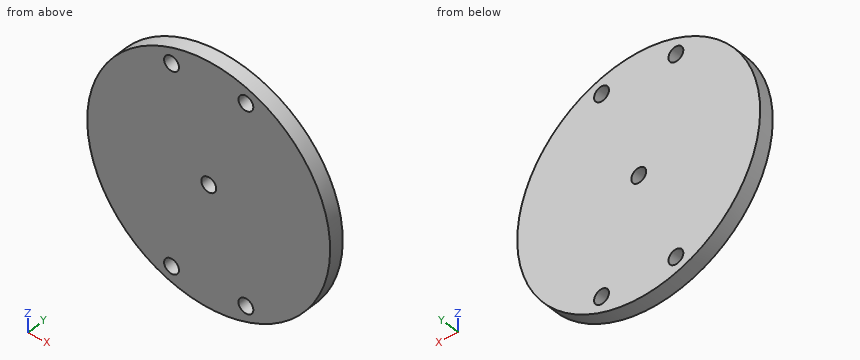
from build123d import *

# Parameters (mm, degrees)
SKETCH1_R           = 49
BOSS_EXTRUDE1_DEPTH = 6
SKETCH2_R           = 3
CUT_EXTRUDE1_DEPTH  = 6


with BuildPart() as part:
    # Sketch1 → Boss-Extrude1 (new body)
    with BuildSketch(Plane(origin=(0, 0, 0), x_dir=(1, 0, 0), z_dir=(0, 1, 0))):
        with Locations(Location((0, 0, 0), (0, 0, 270))):
            Circle(SKETCH1_R)
    extrude(amount=BOSS_EXTRUDE1_DEPTH)

    # Sketch2 → Cut-Extrude1 (cut)
    with BuildSketch(Plane(origin=(0, 6, 0), x_dir=(1, 0, 0), z_dir=(0, 1, 0))):
        with Locations(Location((-15, 40.298883359, 0), (0, 0, 270))):
            Circle(SKETCH2_R)
        with Locations(Location((15, 40.298883359, 0), (0, 0, 270))):
            Circle(SKETCH2_R)
        with Locations(Location((0, 0, 0), (0, 0, 270))):
            Circle(SKETCH2_R)
        with Locations(Location((15, -40.298883359, 0), (0, 0, 270))):
            Circle(SKETCH2_R)
        with Locations(Location((-15, -40.298883359, 0), (0, 0, 270))):
            Circle(SKETCH2_R)
    extrude(amount=-CUT_EXTRUDE1_DEPTH, mode=Mode.SUBTRACT)


solid = part.part
Could you check a few things on this model? Use its own coordinates, in mm. Coordinates: 2 decimals unless noted, no trailing zeros. Order: outer loops, then holes, each group sorted by start corner. A loop starts at its lowest first (then second) coordinate and runs counter-clockwise, first axis right, second up.
Q1. Suppose I cut it at C-C on y = 2.4. Please give me the cut outline in (x, z).
Q2. Will these pins go through, and if not, where does the flat tip stop? pin 1 (2 mm diameter, centred on y = 2, z = 3.5, fed in from +X); pin 2 (5 mm diameter, centred on x = -20, z = 20.5, fed in from -Y); pin 3 (2 mm diameter, centred on x = -13, y = 3.5, fed in from +Z); pin 4 (2 mm diameter, centred on x = -3.5, y = 2, fed in from +Z).
Q3. Suppose I cut it at A-A on x = 0. Please give me the cut outline in (y, z).
Q4. Please list where these lines run through material, in increasing order: L1, parallel to X at y = 2.2, z = -40; L2, parallel to Z at x = -13, y = 5.7; L3, parallel to X at y = 1.15, z = -41.
Q5. Suppose I cut it at D-D on z = 21.5. Please give me the cut outline in (x, y).
Q6. Suppose I cut it at B-B on x = -15. Please give me the cut outline in (y, z), and give its area (3 significant figures).
Answer:
1. outline: circle Ø98 at (0, 0); hole circle Ø6 at (-15, -40.3); hole circle Ø6 at (-15, 40.3); hole circle Ø6 at (0, 0); hole circle Ø6 at (15, -40.3); hole circle Ø6 at (15, 40.3)
2. pin 1: stops at x = 48.94
2. pin 2: stops at y = 0
2. pin 3: stops at z = 47.51
2. pin 4: stops at z = 48.94
3. outline: (0, -49) - (6, -49) - (6, -3) - (0, -3) - close; (0, 3) - (6, 3) - (6, 49) - (0, 49) - close
4. L1: x = -28.3 to -17.99, -12.01 to 12.01, 17.99 to 28.3
4. L2: z = -47.24 to -42.53, -38.06 to 38.06, 42.53 to 47.24
4. L3: x = -26.83 to -17.92, -12.08 to 12.08, 17.92 to 26.83
5. outline: (-44.03, 0) - (44.03, 0) - (44.03, 6) - (-44.03, 6) - close
6. outline: (0, -46.65) - (6, -46.65) - (6, -43.3) - (0, -43.3) - close; (0, -37.3) - (6, -37.3) - (6, 37.3) - (0, 37.3) - close; (0, 43.3) - (6, 43.3) - (6, 46.65) - (0, 46.65) - close
6. area: 488 mm2
